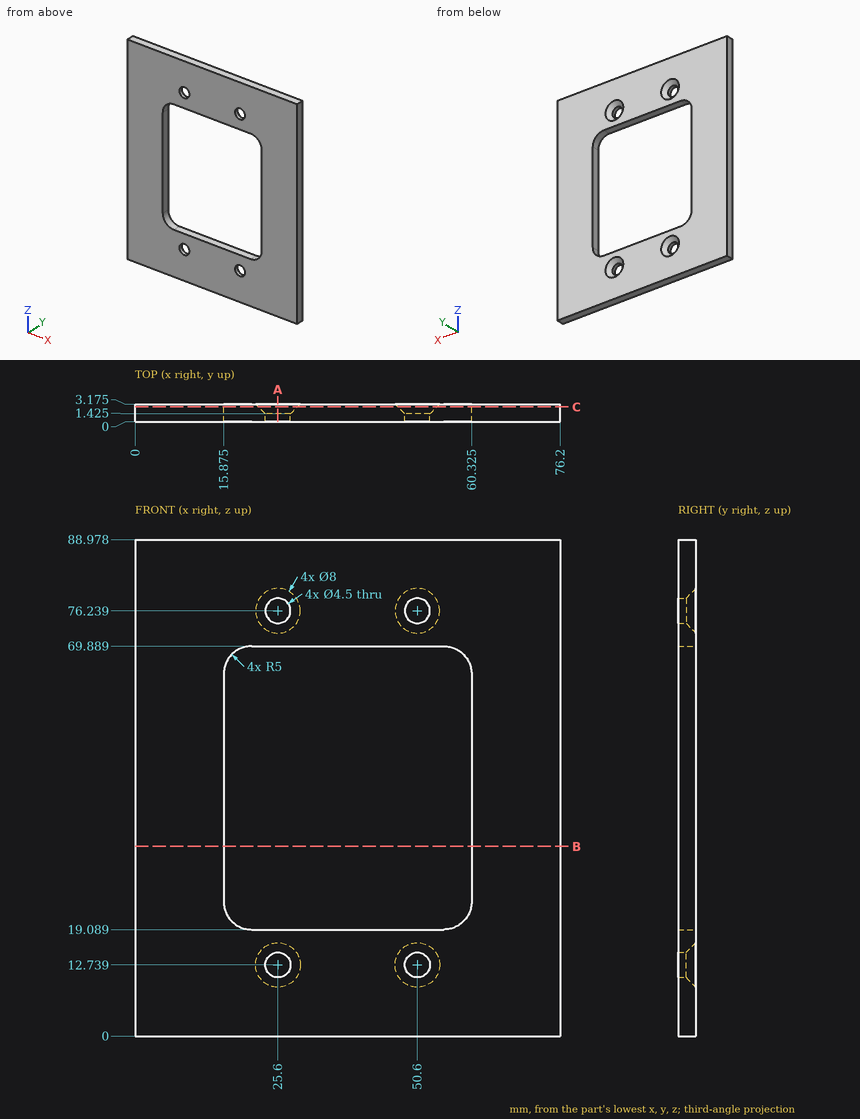
Study the drawing (mm; zero at the part's minimum x, y, z) and answer. Coordinates: 2 decimals unless noted, no trailing zeros. Loops run counter-clockwise (first coordinate to the right, second up) from the corner with the lowest first, then second, coordinate; pieces in that order, holes last. Notation, with made-up numbers: (65, -5.5) -> (79, -5.5) arc R26 cw to (79, 22.5) -> close; hole circle Ø2 at (79.5, 78.5). An arc over 180 degrees is marked (long way). Answer in a Markdown table with one row per item. Add a question column.
1. Consider line 1 (Z direction, x = 25.6, y = 0.95); line 2 (X direction, y = 0.3, z = 30.5) (3 decimals); line 3 (Z direction, x = 52, y = 2.6). Determine where each line is inside the solid, lowest interval first. Write a range as [from, to].
2. The part is cut by section A-A, the plane x = 25.6. Write down the section's boundary in (y, z) (3 decimals).
3. The part is cut by section B-B, the plane z = 34. Write down the section's boundary in (x, y) (3 decimals), then the cut area to 3 significant figures.
4. A flat-ended cylindrical pin translates along its axis: P1, Ø7, axis at x = 25.6, z = 12.739, coming from the +Y side (3 decimals). Find the tip coordinate at first contact, or state that the pin passes through.
5. The part is cut by section C-C, the plane y = 2.65. Write down the section's boundary in (x, z) (3 decimals), then the cut area to 3 significant figures.
Answer below:
| question | item | result |
|---|---|---|
| 1 | line 1 | [0, 10.49], [14.99, 19.09], [69.89, 73.99], [78.49, 88.98] |
| 1 | line 2 | [0, 15.875], [60.325, 76.2] |
| 1 | line 3 | [0, 9.61], [15.86, 19.09], [69.89, 73.11], [79.36, 88.98] |
| 2 | outline | (0, 0) -> (3.175, 0) -> (3.175, 8.739) -> (1.425, 10.489) -> (0, 10.489) -> close; (0, 14.989) -> (1.425, 14.989) -> (3.175, 16.739) -> (3.175, 19.089) -> (0, 19.089) -> close; (0, 69.889) -> (3.175, 69.889) -> (3.175, 72.239) -> (1.425, 73.989) -> (0, 73.989) -> close; (0, 78.489) -> (1.425, 78.489) -> (3.175, 80.239) -> (3.175, 88.978) -> (0, 88.978) -> close |
| 3 | outline | (0, 0) -> (15.875, 0) -> (15.875, 3.175) -> (0, 3.175) -> close; (60.325, 0) -> (76.2, 0) -> (76.2, 3.175) -> (60.325, 3.175) -> close |
| 3 | area | 101 mm2 |
| 4 | P1 | y = 2.675 |
| 5 | outline | (0, 0) -> (76.2, 0) -> (76.2, 88.978) -> (0, 88.978) -> close; hole (15.875, 24.089) arc R5 ccw to (20.875, 19.089) -> (55.325, 19.089) arc R5 ccw to (60.325, 24.089) -> (60.325, 64.889) arc R5 ccw to (55.325, 69.889) -> (20.875, 69.889) arc R5 ccw to (15.875, 64.889) -> close; hole circle Ø6.95 at (25.6, 12.739); hole circle Ø6.95 at (25.6, 76.239); hole circle Ø6.95 at (50.6, 12.739); hole circle Ø6.95 at (50.6, 76.239) |
| 5 | area | 4,390 mm2 |
